```python
from build123d import *

# Parameters (mm, degrees)
F1_DEPTH = 4.3
F0_W     = 129.25
F0_H     = 2
F0_W_2   = 146.25
F2_DEPTH = 10
F3_SIZE  = 3


# Not quite as in the source:
# - a feature names something its author has since deleted; it is built from what else it names


with BuildPart() as f1:
    # F0 (on Top) → F1 (new body)
    with BuildSketch(Plane.XY):
        Polygon((0, 2.85), (0, -2.85), (146.25, -2.85), (146.25, 2.85), (139.25, 2.85), (134.25, 2.85), (5, 2.85), align=None)
        Polygon((-139.25, 2.85), (-146.25, 2.85), (-146.25, -2.85), (0, -2.85), (0, 2.85), (-5, 2.85), (-134.25, 2.85), align=None)
    extrude(amount=F1_DEPTH)

    # F0 (on Top) → F2 (join)
    with BuildSketch(Plane.XY):
        with Locations((69.625, 3.85)):
            Rectangle(F0_W, F0_H)
        with Locations((73.125, -3.85)):
            Rectangle(F0_W_2, F0_H)
        with Locations((-73.125, -3.85)):
            Rectangle(F0_W_2, F0_H)
        with Locations((-69.625, 3.85)):
            Rectangle(F0_W, F0_H)
    extrude(amount=F2_DEPTH)

    # F3
    f3_edges = [f1.edges().sort_by_distance(p)[0] for p in [
        (69.625, 4.85, 0),
    ]]
    chamfer(f3_edges, length=F3_SIZE)


solid = f1.part
```
Source: CAD feature listing. Evaluate the final solid. Frame: model axes, mm. A direction names the side the tool comes from. Round coordinates to 2 decimals unless told otherwise and drop trailing zeros. Order: outer loops, then holes, each group sorted by start corner. A loop starts at its lowest first (then second) coordinate and runs counter-clockwise, first axis right, second up. Notation, with made-up numbers: (21, -7.5) -> (75, -7.5) arc R19 cw to (75, 13.5) -> close; hole circle Ø2 at (16.25, 11). An arc over 180 degrees is marked (long way). One line per item, written item: value. Start each with the question number.
Q1. Material intervals for probe 1 along X at (y, z) = (3.5, 8.75); probe 2 along Y at (x, z) = (-72.5, 5.5); probe 3 along Z at (x, y) = (105.5, -2.5), sorted ascending.
Q2. Pin query (flat end, axial travel): pin 1 (0.6 mm diameter, centred on y = 3.5, z = 3.5, fed in from +X); pin 2 (2 mm diameter, centred on y = 3.5, z = 5.5, fed in from -X); pin 3 (1 mm diameter, centred on x = 2, z = 3, fed in from +Y). Return the tip coordinate at first contact, or that it passes through.
Q3. Section query A-A (z = 6). Return the cut outline in (x, y), plus the area to 3 significant figures.
Q4. Access query for faces 5 (the flat face through (69, 4.85, 6)), 6 (the flat face through (-71, 2.85, 7)). Directions: +Z, -Z, +X, -X, +Y, -Y. A direction counts if a zero-diameter tool reaches every point of the face in a straight line with its end or side. Return the directions, or none.
Q5. Section query C-C (y = -1). Return the cut outline in (x, z).
Q6. Section query B-B (x = 112.5). Return the cut outline in (y, z).
Q7. Draft query along Y for faces 1 (the flat face through (2, -2.85, 7)), 2 (the flat face through (69, 2.85, 7)), 3 (the flat face through (-2, -4.85, 5)), 4 (the flat face through (-71, 4.85, 6)). Return one class per face: pulls with the +Y half, pulls with the -Y half, needs draft (parallel to the pull), parting line crosses it, or undercut.
Findings below:
1. probe 1: -134.25 to -5, 5 to 134.25
1. probe 2: -4.85 to -2.85, 2.85 to 4.85
1. probe 3: 0 to 4.3
2. pin 1: x = 134.25
2. pin 2: x = -134.25
2. pin 3: y = 2.85
3. outline: (-146.25, -4.85) -> (146.25, -4.85) -> (146.25, -2.85) -> (-146.25, -2.85) -> close; (-134.25, 2.85) -> (-5, 2.85) -> (-5, 4.85) -> (-134.25, 4.85) -> close; (5, 2.85) -> (134.25, 2.85) -> (134.25, 4.85) -> (5, 4.85) -> close
3. area: 1,100 mm²
4. face 5: +Z, -Z, +X, -X, +Y
4. face 6: +Z, +X, -X
5. outline: (-146.25, 0) -> (146.25, 0) -> (146.25, 4.3) -> (-146.25, 4.3) -> close
6. outline: (-4.85, 0) -> (1.85, 0) -> (4.85, 3) -> (4.85, 10) -> (2.85, 10) -> (2.85, 4.3) -> (-2.85, 4.3) -> (-2.85, 10) -> (-4.85, 10) -> close
7. face 1: undercut
7. face 2: undercut
7. face 3: pulls with the -Y half
7. face 4: pulls with the +Y half
